Could you check a few things on this model? Use its own coordinates, in mm. A direction names the side the tool comes from. Coordinates: 2 decimals unless noted, no trailing zeros. Loops run counter-clockwise (first coordinate to the right, second up) from the corner with the lowest first, then second, coordinate; pieces in that order, holes last. Notation, with made-up numbers: (47, -24) -> (88, -24) arc R10 cw to (88, -19) -> close; hole circle Ø7 at (-31.5, 24). An arc over 180 degrees is marked (long way). One line per question, with ' | ' between items.
from build123d import *

# Parameters (mm, degrees)
BASE_FLANGE1_DEPTH = 3.175


# Sheet-metal steps are written as plain solids
with BuildPart() as part:
    # Sketch1 → Base-Flange1 (new body)
    with BuildSketch(Plane(origin=(0, 0, 0), x_dir=(1, 0, 0), z_dir=(0, 1, 0))):
        with BuildLine():
            Line((-29.887299957, -182.597941739), (-32.985733317, -146.952874795))
            Line((-32.985733317, -146.952874795), (-32.985733317, -94.571650999))
            Line((-32.985733317, -94.571650999), (-46.087855458, -48.292438117))
            ThreePointArc((-46.087855458, -48.292438117), (-43.944076056, -42.701188324), (-37.974785272, -43.175985032))
            ThreePointArc((-37.974785272, -43.175985032), (0, -57.5), (37.974785272, -43.175985032))
            ThreePointArc((37.974785272, -43.175985032), (43.944076056, -42.701188324), (46.087855458, -48.292438117))
            Line((46.087855458, -48.292438117), (32.985733317, -94.571650999))
            Line((32.985733317, -94.571650999), (32.985733317, -146.952874795))
            Line((32.985733317, -146.952874795), (29.887299957, -182.597941739))
            ThreePointArc((29.887299957, -182.597941739), (0, -210), (-29.887299957, -182.597941739))
        make_face()
    extrude(amount=-BASE_FLANGE1_DEPTH)


solid = part.part
1) If we section it at D-D on x = 2: Please give me the cut outline in (y, z) (3 decimals), and give its area (3 significant figures).
Data:
outline: (-3.175, 57.465) -> (0, 57.465) -> (0, 209.933) -> (-3.175, 209.933) -> close | area: 484 mm²
2) I need wall thicknesses on line 1 along X through (y, z) = (-1.25, 123); line 2 along X through (y, z) = (-0.3, 163); line 3 along Z through (x, y) = (21.5, -1.75). Which ranges of each line are inside material? Lowest first, please. Write a range as from..to.
Data:
line 1: -32.99..32.99 | line 2: -31.59..31.59 | line 3: 53.33..200.92
3) On a 3-axis mill with a long thin cutter (end or side, diameter ignored), from which of +Z, -Z, +X, -X, +Y, -Y can I reach the whole of each face in a straight line? I mean faces 4 (the face through (-0.581, -1.565, 57.497)), 5 (the face through (-32.986, -2, 121)). Say none if no direction works.
Data:
face 4: -Z, +Y, -Y | face 5: +Z, -X, +Y, -Y
4) If we section it at B-B on y = -1.3: Please give me the cut outline in (x, z), and give its area (3 significant figures).
Data:
outline: (-46.09, 48.29) arc R5 ccw to (-37.97, 43.18) arc R57.5 cw to (37.97, 43.18) arc R5 ccw to (46.09, 48.29) -> (32.99, 94.57) -> (32.99, 146.95) -> (29.89, 182.6) arc R30 ccw to (-29.89, 182.6) -> (-32.99, 146.95) -> (-32.99, 94.57) -> close | area: 10,300 mm²
5) We'd pull the mould along X, two halves only. Please class faces 1 (the face through (32.986, -2, 120)), 2 (the face through (1, 0, 125)), 3 (the face through (43.868, -1.565, 42.654)): pulls with the +X half, pulls with the -X half, needs draft (parallel to the pull), parting line crosses it, or undercut.
Data:
face 1: pulls with the +X half | face 2: needs draft | face 3: undercut
6) If we section it at C-C on z = 106: Please give me the cut outline in (x, y) (3 decimals).
Data:
outline: (-32.986, -3.175) -> (32.986, -3.175) -> (32.986, 0) -> (-32.986, 0) -> close
7) If we section it at A-A on z = 55: Please give me the cut outline in (x, y) (1 decimal), and give its area (3 significant figures).
Data:
outline: (-44.2, -3.2) -> (-16.8, -3.2) -> (-16.8, 0) -> (-44.2, 0) -> close; (16.8, -3.2) -> (44.2, -3.2) -> (44.2, 0) -> (16.8, 0) -> close | area: 174 mm²
8) I'm going to push flat-ended pins straight in: pin 1 Ø8 at (x, z) = (-23.5, 92.5) entering from +Y; pin 2 Ø1 at (y, z) = (-3, 176.5) entering from +X. Where does each tip first touch, or does it pass through?
Data:
pin 1: y = 0 | pin 2: x = 30.46
